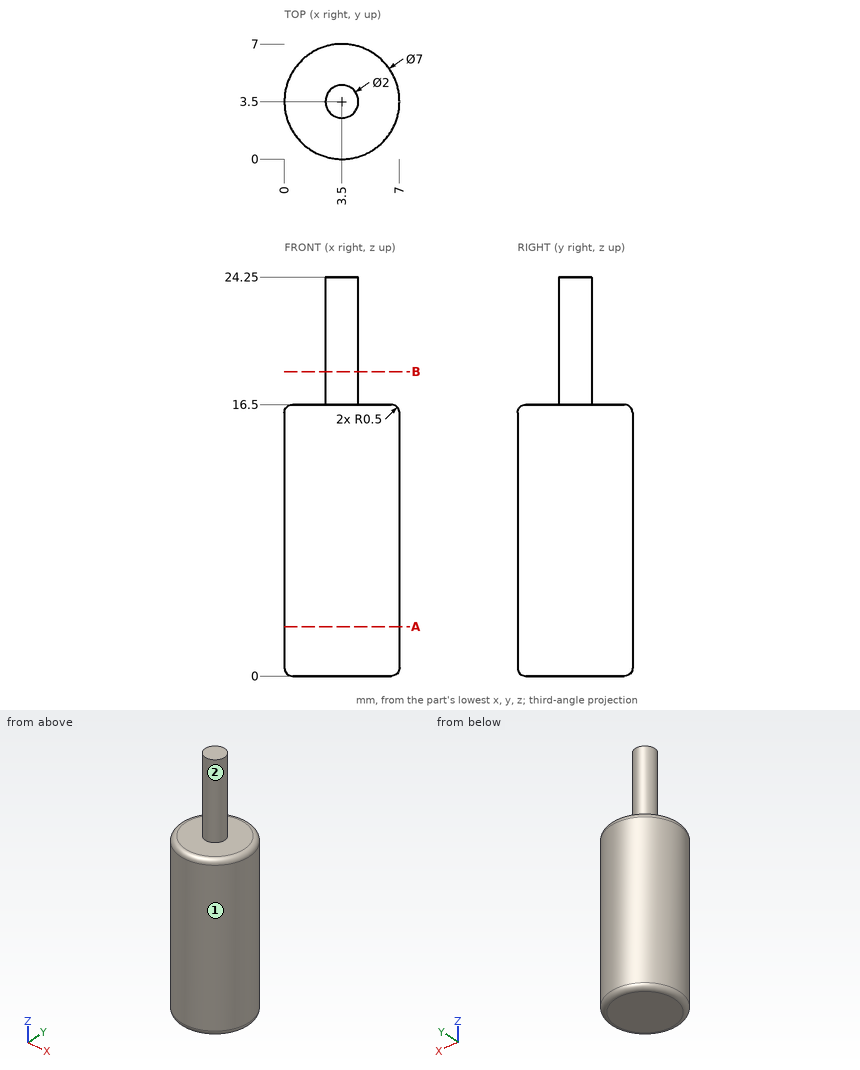
Source: three-view drawing plus pictorial views. Frame: mm from the lowest corner of the part. A direction names the side the tool comes from. Give positions to 0.01 mm unless a question says otherwise; leave off trailing zeros. Loops run counter-clockwise (first coordinate to the right, second up) from the corner with the lowest first, then second, coordinate; pieces in that order, holes last. Notation, with made-up numbers: (-8.5, 79) -> (0.5, 79) arc R36 cw to (0.5, 118) -> close; hole circle Ø3 at (-8.75, 64). An arc over 180 degrees is marked (long way). Put each result on its own line as item: value. Start each with the question number.
1) Reachability of the marked faces 1 and 2 from +Z, -Z, +X, -X, +Y, -Y: full face, straight path, thin tool, end or side. Return the list, or none.
2) Contact query for flat-ended pins moving along their axis: P1, Ø1.5, axis at x = 4.5, z = 14.5, coming from the +Y side; P2, Ø1, axis at x = 4.5, z = 19.5, coming from the +Y side; P3, Ø2, axis at y = 5.5, z = 8, coming from the +X side. Output: stop coordinate, or through.
3) Cut plane B-B (z = 18.5). Return loops of the section in (x, y).
4) Cut plane A-A (z = 3). Return loops of the section in (x, y).
5) Material intervals for probe 1 along Z at (x, y) = (4, 5.75); probe 2 along Y at (x, z) = (0.75, 8.75); probe 3 along X at (y, z) = (2.25, 16.25), sorted ascending.
Results are:
1. face 1: +Z, -Z
1. face 2: +Z
2. P1: stops at y = 6.99
2. P2: stops at y = 4.37
2. P3: stops at x = 6.85
3. outline: circle Ø2 at (3.5, 3.5)
4. outline: circle Ø7 at (3.5, 3.5)
5. probe 1: z = 0 to 16.5
5. probe 2: y = 1.33 to 5.67
5. probe 3: x = 0.3 to 6.7
